Geometry check sheet. Reference: the model listing, model coordinates, mm. A direction names the side the tool comes from. Coordinates: 2 decimals unless noted, no trailing zeros. Write each loop counter-clockwise with the first axis right and the second up, starting at its lowest first coordinate (ties: lowest second). Pieces come first, ordered by that corner, then holes. Notation, with made-up numbers: M -19.75,-23.75 L 0.25,-23.75 A32 cw 0.25,15.25 Z; hole C -9.5,36 d1. An arc over 180 degrees is marked long. Write each question's results on one line, items separated by ' | '.
```python
from build123d import *

# Parameters (mm, degrees)
F0_W     = 70
F0_H     = 90
F1_DEPTH = 35
F2_T     = -2
F3_R     = 3.5
F4_DEPTH = 4
F5_W     = 20
F5_H     = 10
F5_W_2   = 15
F5_H_2   = 6
F6_DEPTH = 2
F7_W     = 10
F7_H     = 10
F8_DEPTH = 2


with BuildPart() as f1:
    # F0 (on Top) → F1 (new body)
    with BuildSketch(Plane.XY):
        Rectangle(F0_W, F0_H)
    extrude(amount=F1_DEPTH)

    # F2
    f2_openings = [f1.faces().sort_by_distance(p)[0] for p in [
        (0, 0, 35),
    ]]
    offset(amount=F2_T, openings=f2_openings)

    # F3 (on face) → F4 (join)
    with BuildSketch(Plane.XY.offset(2)):
        with Locations((-27.5, 37.5)):
            Circle(F3_R)
        with Locations((27.5, -37.5)):
            Circle(F3_R)
        with Locations((27.5, 37.5)):
            Circle(F3_R)
        with Locations((-27.5, -37.5)):
            Circle(F3_R)
    extrude(amount=F4_DEPTH)

    # F5 (on face) → F6 (cut, through all)
    with BuildSketch(Plane.XZ.offset(45)):
        with Locations((-20, 12)):
            Rectangle(F5_W, F5_H)
        with Locations((18.5, 18)):
            Rectangle(F5_W_2, F5_H_2)
    extrude(amount=-F6_DEPTH, mode=Mode.SUBTRACT)

    # F7 (on face) → F8 (cut, through all)
    with BuildSketch(Plane(origin=(0, 45, 0), x_dir=(-1, 0, 0), z_dir=(0, 1, 0))):
        with Locations((-2, 10)):
            Rectangle(F7_W, F7_H)
    extrude(amount=-F8_DEPTH, mode=Mode.SUBTRACT)


solid = f1.part
```
Q1. Sectioned sample at B-B on x = 5.5. Record the cut outline in (y, z), and give its area (3 significant figures).
Geometry check:
outline: M -45,0 L 45,0 L 45,5 L 43,5 L 43,2 L -43,2 L -43,35 L -45,35 Z; M 43,15 L 45,15 L 45,35 L 43,35 Z | area: 292 mm2
Q2. Sectioned sample at A-A on z = 3. Record the cut outline in (x, y), and give its area (3 significant figures).
Geometry check:
outline: M -35,-45 L 35,-45 L 35,45 L -35,45 Z; C -27.5,-37.5 d7; C -27.5,37.5 d7; C 27.5,-37.5 d7; C 27.5,37.5 d7; hole M -33,-43 L 33,-43 L 33,43 L -33,43 Z | area: 778 mm2
Q3. Depth check by flat-ended pin: P1, Ø7.5, axis at x = -28, y = -37, coming from the +Z side; P2, Ø1.5, axis at x = -3.5, y = -7.5, coming from the +Z side. Enter the tip coordinate at first touch or a pass-through.
Geometry check:
P1: stops at z = 6 | P2: stops at z = 2
Q4. Sectioned sample at C-C on z = 31. Record the cut outline in (x, y).
Geometry check:
outline: M -35,-45 L 35,-45 L 35,45 L -35,45 Z; hole M -33,-43 L 33,-43 L 33,43 L -33,43 Z
Q5. Mould release check, pull along Z, two halves, no side actions. Record for faces 4 (the flat face through (0, 45, 17)), 5 (the flat face through (27, 38, 6)), 6 (the flat face through (-3, 44, 10)): pulls with the +Z half, pulls with the -Z half, needs draft (parallel to the pull), parting line crosses it, or undercut.
Geometry check:
face 4: needs draft | face 5: pulls with the +Z half | face 6: undercut
Q6. Access from +Z, -Z, +X, -X, +Y, -Y to the whole of each face (thin tool, end or side, straight path). Record for faces 1 (the flat face through (18, -44, 21)), 2 (the flat face through (-33, -1, 18)), 3 (the flat face through (7, 44, 10)).
Geometry check:
face 1: -Y | face 2: +Z | face 3: +Y
Q7. Scan lines: probe 1 along Y at (x, z) = (8.5, 13); probe 2 along X at (y, z) = (31, 32); probe 3 along Z at (x, y) = (-28, 27). Record each from-to range of solid material in increasing order.
Geometry check:
probe 1: y = -45 to -43, 43 to 45 | probe 2: x = -35 to -33, 33 to 35 | probe 3: z = 0 to 2
Q8. Sectioned sample at D-D on y = 28. Record the cut outline in (x, z).
Geometry check:
outline: M -35,0 L 35,0 L 35,35 L 33,35 L 33,2 L -33,2 L -33,35 L -35,35 Z
